from build123d import *

# Parameters (mm, degrees)
ESQUISSE1_R           = 4
BOSS_EXTRU_1_DEPTH    = 14
CHANFREIN1_SIZE       = 0.5
TROU_TARAUD_M41_D     = 3.3
TROU_TARAUD_M41_DEPTH = 11.5
TROU_TARAUD_M41_TIP   = 0.991420021


with BuildPart() as part:
    # Esquisse1 → Boss.-Extru.1 (new body)
    with BuildSketch(Plane.XY):
        Circle(ESQUISSE1_R)
    extrude(amount=BOSS_EXTRU_1_DEPTH)

    # Chanfrein1
    chanfrein1_edges = [part.edges().sort_by_distance(p)[0] for p in [
        (-4, 0, 14),
    ]]
    chamfer(chanfrein1_edges, length=CHANFREIN1_SIZE)

    # Trou taraudé M41
    with Locations(Plane(origin=(0, 0, 0), x_dir=(-1, 0, 0), z_dir=(0, 0, -1))):
        with Locations((0, 0)):
            Hole(TROU_TARAUD_M41_D / 2, depth=TROU_TARAUD_M41_DEPTH)
            with Locations((0, 0, -(TROU_TARAUD_M41_DEPTH + TROU_TARAUD_M41_TIP / 2))):  # 118° drill point
                Cone(0, TROU_TARAUD_M41_D / 2, TROU_TARAUD_M41_TIP, mode=Mode.SUBTRACT)


solid = part.part
Design review of the part built by this model. Coordinates are the model's own, in mm. A direction names the side the tool comes from. Coordinates: 2 decimals unless noted, no trailing zeros. Loops run counter-clockwise (first coordinate to the right, second up) from the corner with the lowest first, then second, coordinate; pieces in that order, holes last. Notation, with made-up numbers: (35, -38.75) - (53, -38.75) arc R15 cw to (53, -11.75) - close; hole circle Ø11 at (24.5, 24). An arc over 180 degrees is marked (long way). Use CSV: the item, a comma, the result in double quotes. Start each with the question number.
1. For faces 1 (the cylindrical face through (-1.216, 1.115, 5.831)), 2 (the flat face through (2, 0, 0)), list the 3-axis set-ups (+Z, -Z, +X, -X, +Y, -Y) from which the entire face can be reached by the end or side of a thin tool; tool diameter is ignored.
2. Clearance check with flat-ended pins moving along their axes: pin 1 (2 mm diameter, centred on y = -2.5, z = 9, fed in from -X); pin 2 (2 mm diameter, centred on x = -0.5, y = 0, fed in from -Z); pin 3 (3 mm diameter, centred on y = -0.5, z = 2, fed in from +X); pin 4 (1 mm diameter, centred on y = -2, z = 10, fed in from +X). State where each tip first meets the part, or that it passes through.
3. Add section A-A on z = 5.5. Give the boundary of the cut face in (x, y), plus the area to 3 significant figures.
4. To check wall thickness, follow probe 1 along Y at (x, z) = (0, 6.25); probe 2 along X at (y, z) = (-0.5, 4); probe 3 along Y at (x, z) = (-1, 8.75). State the ranges of each line that lie inside material, in increasing order.
Resolved:
1,face 1,"-Z"
1,face 2,"-Z, +X, -X, +Y, -Y"
2,pin 1,"x = -3.71"
2,pin 2,"z = 11.59"
2,pin 3,"x = 4"
2,pin 4,"x = 3.71"
3,outline,"circle Ø8 at (0, 0); hole circle Ø3.3 at (0, 0)"
3,area,"41.7 mm2"
4,probe 1,"-4 to -1.65, 1.65 to 4"
4,probe 2,"-3.97 to -1.57, 1.57 to 3.97"
4,probe 3,"-3.87 to -1.31, 1.31 to 3.87"
